Geometry check sheet. Reference: the model listing, model coordinates, mm. Coordinates: 2 decimals unless noted, no trailing zeros. Write each loop counter-clockwise with the first axis right and the second up, starting at its lowest first coordinate (ties: lowest second). Pieces come first, ordered by that corner, then holes. Notation, with made-up numbers: (20.25, 28) -> (36.25, 28) arc R18 cw to (36.25, 54) -> close; hole circle Ø7 at (9, 64). An arc over 180 degrees is marked (long way). Use a Markdown table: item, result.
Autodesk Inventor part; units mm, degrees
ref_plane "YZ Plane" through (0, 0, 0) normal (1, 0, 0) x (0, 1, 0)
ref_plane "XZ Plane" through (0, 0, 0) normal (0, 1, 0) x (-1, 0, 0)
ref_plane "XY Plane" through (0, 0, 0) normal (0, 0, 1) x (1, 0, 0)
sketch "Sketch1" plane through (0, 0, 0) normal (0, 0, 1) x (1, 0, 0)
  circle A0 centre (0, 0) radius 5.644444
  dimension "d0" = 11.28889
extrude "Extrusion1" add sketch "Sketch1" against normal blind 11.288889 draft -10
sketch "Sketch3" plane through (0, 0, 0) normal (0, 0, 1) x (1, 0, 0)
  circle A0 centre (0, 0) radius 3.653909
  line L0 (-14.2875, 0) -> (-7.14375, 12.373338)
  line L1 (-7.14375, 12.373338) -> (7.14375, 12.373338)
  line L2 (7.14375, 12.373338) -> (14.2875, 0)
  line L3 (14.2875, 0) -> (7.14375, -12.373338)
  line L4 (7.14375, -12.373338) -> (-7.14375, -12.373338)
  line L5 (-7.14375, -12.373338) -> (-14.2875, 0)
  line L6 (0, 0) -> (-14.2875, 0) construction
  dimension "d11" = 28.575
sketch "Sketch3 outline for Extrusion3" plane through (0, 0, 0) normal (0, 0, 1) x (1, 0, 0)
  line L0 (-14.2875, 0) -> (-7.14375, 12.373338)
  line L1 (-7.14375, 12.373338) -> (7.14375, 12.373338)
  line L2 (7.14375, 12.373338) -> (14.2875, 0)
  line L3 (14.2875, 0) -> (7.14375, -12.373338)
  line L4 (7.14375, -12.373338) -> (-7.14375, -12.373338)
  line L5 (-7.14375, -12.373338) -> (-14.2875, 0)
extrude "Extrusion3" add sketch "Sketch3 outline for Extrusion3" along normal blind 3.175 draft -10
properties part number "Driven Pin"
Item 1: Thickness scan on L1, parallel to Z at x = -2, y = -9.5 (3 decimals); L2, parallel to X at y = -9.5, z = 1; L3, parallel to Y at x = -0.5, z = -4.75. Record the ranges inside material, lowest first. Write a range as [from, to].
Answer block:
| item | result |
|---|---|
| L1 | z = [0, 3.175] |
| L2 | x = [-8.6, 8.6] |
| L3 | y = [-4.78, 4.78] |
Item 2: Depth check by flat-ended pin: P1, Ø2, axis at y = -5, z = -4, coming from the -X side; P2, Ø3, axis at x = -2.5, z = -5.5, coming from the -Y side; P3, Ø4, axis at x = 11, z = 0, coming from the +Y side. Enter the tip coordinate at first touch or a pass-through.
Answer block:
| item | result |
|---|---|
| P1 | stops at x = -2.93 |
| P2 | stops at y = -4.66 |
| P3 | stops at y = 9.16 |
Item 3: Section check C-C on y = -10. Record the boundary of the cut face in (x, z) (3 decimals), then the cut area to 3 significant figures.
Answer block:
| item | result |
|---|---|
| outline | (-8.514, 0) -> (8.514, 0) -> (7.868, 3.175) -> (-7.868, 3.175) -> close |
| area | 52.0 mm^2 |
Item 4: Section check D-D on y = -7.5. Record the boundary of the cut face in (x, z) (3 decimals).
Answer block:
| item | result |
|---|---|
| outline | (-9.957, 0) -> (9.957, 0) -> (9.311, 3.175) -> (-9.311, 3.175) -> close |
Item 5: Section check A-A on x = 0. Record the boundary of the cut face in (y, z) (1 decimal), then the cut area to 3 significant figures.
Answer block:
| item | result |
|---|---|
| outline | (-12.4, 0) -> (-5.6, 0) -> (-3.7, -11.3) -> (3.7, -11.3) -> (5.6, 0) -> (12.4, 0) -> (11.8, 3.2) -> (-11.8, 3.2) -> close |
| area | 182 mm^2 |
Item 6: Section check B-B on z = 0.75. Record the boundary of the cut face in (x, y).
Answer block:
| item | result |
|---|---|
| outline | (-14.13, 0) -> (-7.07, -12.24) -> (7.07, -12.24) -> (14.13, 0) -> (7.07, 12.24) -> (-7.07, 12.24) -> close |
Item 7: Mould release check, pull along X, two halves, no side actions. Record for faces 1 (the flat face through (-10.527, 5.962, 1.565)), 2 (the flat face through (10.527, -5.962, 1.565)), 3 (the flat face through (0, 6, 0)), 4 (the conical face through (-0.963, -4.336, -6.82)): +X half, -X half, draft (parallel to the pull), parting line (faces both ways), or undercut.
Answer block:
| item | result |
|---|---|
| face 1 | -X half |
| face 2 | +X half |
| face 3 | draft |
| face 4 | parting line |
